from build123d import *

# Parameters (mm, degrees)
F1_DEPTH = 125
F3_DEPTH = 3
F5_DEPTH = 3


with BuildPart() as f1:
    # F0 (on Front) → F1 (new body, symmetric)
    with BuildSketch(Plane.XZ):
        with BuildLine():
            Line((-9.569632, 7), (-11.569632, 7))
            ThreePointArc((-11.569632, 7), (-4.569632, 0), (2.430368, 7))
            Line((2.430368, 7), (0.430368, 7))
            ThreePointArc((0.430368, 7), (-4.569632, 2), (-9.569632, 7))
        make_face()
    extrude(amount=F1_DEPTH, both=True)

    # F2 (on face) → F3 (join)
    with BuildSketch(Plane.XZ.offset(125)):
        with BuildLine():
            Line((0.430368, 7), (-9.569632, 7))
            ThreePointArc((-9.569632, 7), (-4.569632, 2), (0.430368, 7))
        make_face()
    extrude(amount=-F3_DEPTH)

    # F4 (on face) → F5 (join)
    with BuildSketch(Plane(origin=(0, 125, 0), x_dir=(-1, 0, 0), z_dir=(0, 1, 0))):
        with BuildLine():
            Line((9.569632, 7), (-0.430368, 7))
            ThreePointArc((-0.430368, 7), (4.569632, 2), (9.569632, 7))
        make_face()
    extrude(amount=-F5_DEPTH)


solid = f1.part
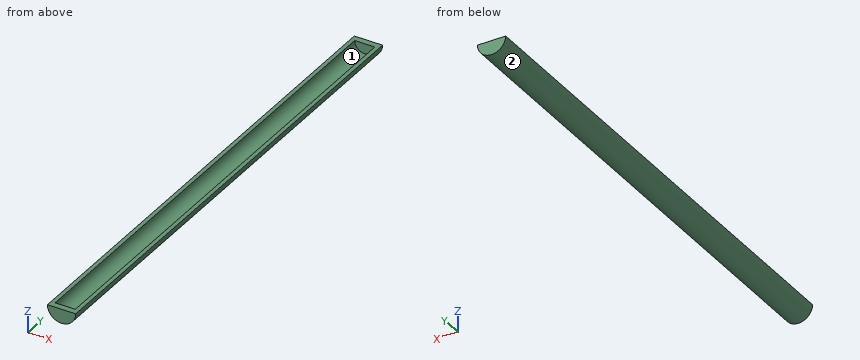
For this review, take the finished solid that the model builds, in its own axes (mm). Face numbers are marked on the shaded views. A direction names the side the tool comes from. Round coordinates to 2 decimals unless told otherwise and drop trailing zeros. Write each loop counter-clockwise with the first axis right and the second up, starting at its lowest first coordinate (ties: lowest second). Pieces come first, ordered by that corner, then holes. Notation, with made-up numbers: M 39.5,-5 L 44.5,-5 A25 cw 44.5,17 Z; hole C -13,70 d8. An arc over 180 degrees is marked long. Write item = value, one per line. Start each with the question number.
(1) For line 1 along Y through (x, z) = (-0.75, 6.5); line 2 along X through (y, z) = (-92, 3.5); line 3 along X through (y, z) = (26.5, 6), list the stretches that pass through material, from the lowest coordinate up.
(2) For the marked faces 1 and 2, list the 3-axis set-ups (+Z, -Z, +X, -X, +Y, -Y) from which the entire face can be reached by the end or side of a thin tool; tool diameter is ignored.
(3) Clearance check with flat-ended pins moving along their axes: pin 1 Ø5 at (x, y) = (-8, -63) entering from -Z; pin 2 Ø2 at (x, y) = (-1.5, 93.5) entering from +Z; pin 3 Ø1 at (x, y) = (-2, 59.5) entering from +Z. State where each tip first meets the part, or that it passes through.
(4) We need section B-B (x = -7). Give the boundary of the cut face in (y, z).
(5) We need section C-C (y = -105.5). Give the boundary of the cut face in (x, z).
(6) We need section A-A (z = 4.25). Give the boundary of the cut face in (x, y).
Results found:
q1.line_1 = -125 to -122, 122 to 125
q1.line_2 = -10.63 to -8.14, -1 to 1.49
q1.line_3 = -11.5 to -9.47, 0.33 to 2.36
q2.face_1 = +Z
q2.face_2 = -Z, +Y, -Y
q3.pin_1 = 0.06
q3.pin_2 = 4.1
q3.pin_3 = 3.05
q4.outline = M -125,0.44 L 125,0.44 L 125,7 L 122,7 L 122,2.63 L -122,2.63 L -122,7 L -125,7 Z
q5.outline = M -11.57,7 A7 ccw 2.43,7 L 0.43,7 A5 cw -9.57,7 Z
q6.outline = M -11.01,-125 L 1.87,-125 L 1.87,125 L -11.01,125 Z; hole M -8.75,-122 L -0.39,-122 L -0.39,122 L -8.75,122 Z
